Model file for the job. Use its own axes, mm. A direction names the side the tool comes from. Give positions to 0.01 mm unless a question says otherwise; leave off trailing zeros. Order: outer loops, then holes, each group sorted by start corner. A loop starts at its lowest first (then second) coordinate and runs counter-clockwise, first axis right, second up. Notation, with made-up numbers: (63, 17) - (115, 17) arc R8 cw to (115, 23) - close; hole circle Ø4 at (50.5, 61). An arc over 180 degrees is marked (long way). Use CSV: the item, a comma, the result in double quotes. Start each with the question number.
(1) Tool access for faces 1 (the flat face through (13, 0, 12)), 2 (the flat face through (10.92, 27.56, 12.7)): list every direction of +Z, -Z, +X, -X, +Y, -Y with a clear straight run to the whole face (end or side of a thin tool).
(2) Drop flat-ended pins along their axis: pin 1 Ø1.5 at (x, z) = (10.5, 14.5) entering from +Y; pin 2 Ø3 at (y, z) = (39.5, 18.5) entering from +X; pin 3 Ø4 at (x, y) = (8.5, 36) entering from -Z; pin 4 Ø4 at (x, z) = (19.5, 16.5) entering from +Y. Give the stop position or say it passes through.
(3) Pull direction Y, two halves, no side cores. Call faces 3 (the flat face through (6.16, 35.81, 12.7)), 4 (the flat face through (10, 18, 0)), 5 (the flat face through (26.058, 1.571, 12.698)), 6 (the flat face through (17.27, 16.56, 12.7)): +Y half, -Y half, draft (parallel to the pull), parting line (faces both ways), or undercut.
(4) Band-saw the part on C-C, the plane y = 24. Give the cut face in (x, z), then the cut area to 3 significant figures.
(5) Band-saw the part on B-B, the plane y = 28.5. Give the cut face in (x, z).
(6) Probe L1, parallel to Y at x = 16, z = 6.25; L2, parallel to X at y = 21, z = 14.5; L3, parallel to Y at x = 11, z = 10.5. List the from-to ranges inside material, lowest first.
from build123d import *

# Parameters (mm, degrees)
BOSS_EXTRUDE1_DEPTH = 25.0444
CUT_EXTRUDE1_DEPTH  = 58.602407639
LPATTERN1_COUNT     = 17
LPATTERN1_PITCH     = 3.175


with BuildPart() as part:
    # Sketch1 → Boss-Extrude1 (new body)
    with BuildSketch(Plane.XY):
        Polygon((0, 42.926), (0, 0), (25.908, 0), (26.917900092, 2.319009706), (2.655725985, 44.342327962), align=None)
    extrude(amount=BOSS_EXTRUDE1_DEPTH)

    # Sketch2 → Cut-Extrude1 (cut, through all)
    with BuildSketch(Plane.XY.offset(25.0444)):
        Polygon((2.655725985, 44.342327962), (1.766174751, 41.030721161), (4.243225985, 41.592697305), align=None)
    cut_extrude1 = extrude(amount=-CUT_EXTRUDE1_DEPTH, mode=Mode.SUBTRACT)

    # LPattern1: Cut-Extrude1 ×17
    with Locations(*[Vector(0.5000000000000007, -0.8660254037844384, 0) * (i * LPATTERN1_PITCH) for i in range(1, LPATTERN1_COUNT)]):
        add(cut_extrude1, mode=Mode.SUBTRACT)


solid = part.part
Answer block:
1,face 1,"+Z, -Z, +X, -X, -Y"
1,face 2,"+Z, -Z"
2,pin 1,"stops at y = 30.59"
2,pin 2,"stops at x = 5.83"
2,pin 3,"stops at z = 0"
2,pin 4,"stops at y = 16.85"
3,face 3,"undercut"
3,face 4,"draft"
3,face 5,"-Y half"
3,face 6,"undercut"
4,outline,"(0, 0) - (13.47, 0) - (13.47, 25.04) - (0, 25.04) - close"
4,area,"337 mm2"
5,outline,"(0, 0) - (10.03, 0) - (10.03, 25.04) - (0, 25.04) - close"
6,L1,"y = 0 to 19.38"
6,L2,"x = 0 to 14.99"
6,L3,"y = 0 to 27.58"
